```python
from build123d import *

# Parameters (mm, degrees)
EXTRUDE_1_DEPTH     = 35
SKETCH_7_W          = 12
SKETCH_7_H          = 6.5
EXTRUDE_3_DEPTH     = 4
CUT_EXTRUDE_1_REACH = 5
SKETCH_2_R          = 1.5
CUT_EXTRUDE_2_DEPTH = 28.8
SKETCH_6_W          = 12
SKETCH_6_H          = 5.977376498
SKETCH_6_R          = 1.5
EXTRUDE_2_DEPTH     = 4
CUT_EXTRUDE_3_REACH = 29.964
SKETCH_9_R          = 1.5
FILLET_1_R          = 3
FILLET_2_R          = 2
MM_CLEARANCE_1_D    = 3


with BuildPart() as part:
    # 草图1 → 凸台-拉伸1 (new body)
    with BuildSketch(Plane.XY):
        Polygon((-25.8, 21.661752689), (-25.8, -6.245255474), (3, -6.245255474), (3, 21.718248175), (0, 21.718248175), (0, -3.245255474), (-22.8, -3.245255474), (-22.8, 21.718248175), (-25.8, 21.718248175), align=None)
    extrude(amount=EXTRUDE_1_DEPTH)

    # 草图7 → 凸台-拉伸3 (add)
    with BuildSketch(Plane(origin=(0, -3.245255474, 0), x_dir=(1, 0, 0), z_dir=(0, 1, 0))):
        with Locations((-11.4, -3.272623502)):
            Rectangle(SKETCH_7_W, SKETCH_7_H)
    extrude(amount=EXTRUDE_3_DEPTH)

    # 草图2 → 切除-拉伸1 (cut, up to next)
    with BuildSketch(Plane(origin=(0, -3.245255474, 0), x_dir=(1, 0, 0), z_dir=(0, 1, 0)), mode=Mode.PRIVATE) as cut_extrude_1_sk1:
        with Locations((-11.4, -4.329564509)):
            Circle(SKETCH_2_R)
    cut_extrude_1_tool1 = extrude(cut_extrude_1_sk1.sketch, amount=-CUT_EXTRUDE_1_REACH, mode=Mode.PRIVATE) & part.part
    add(cut_extrude_1_tool1.solids().sort_by_distance((-11.4, -3.245255, 4.329565))[0], mode=Mode.SUBTRACT)
    # 草图2 → 切除-拉伸1 (cut, up to next)
    with BuildSketch(Plane(origin=(0, -3.245255474, 0), x_dir=(1, 0, 0), z_dir=(0, 1, 0)), mode=Mode.PRIVATE) as cut_extrude_1_sk2:
        with Locations((-11.4, -31.529564509)):
            Circle(SKETCH_2_R)
    cut_extrude_1_tool2 = extrude(cut_extrude_1_sk2.sketch, amount=-CUT_EXTRUDE_1_REACH, mode=Mode.PRIVATE) & part.part
    add(cut_extrude_1_tool2.solids().sort_by_distance((-11.4, -3.245255, 31.529565))[0], mode=Mode.SUBTRACT)
    # 草图2 → 切除-拉伸1 (cut, up to next)
    with BuildSketch(Plane(origin=(0, -3.245255474, 0), x_dir=(1, 0, 0), z_dir=(0, 1, 0)), mode=Mode.PRIVATE) as cut_extrude_1_sk3:
        with BuildLine():
            Line((-14.65, -18), (-14.65, -16.99341649))
            ThreePointArc((-14.65, -16.99341649), (-11.4, -6.5), (-8.15, -16.99341649))
            Line((-8.15, -16.99341649), (-8.15, -18))
            ThreePointArc((-8.15, -18), (-11.4, -21.25), (-14.65, -18))
        make_face()
    cut_extrude_1_tool3 = extrude(cut_extrude_1_sk3.sketch, amount=-CUT_EXTRUDE_1_REACH, mode=Mode.PRIVATE) & part.part
    add(cut_extrude_1_tool3.solids().sort_by_distance((-11.4, -3.245255, 13.308508))[0], mode=Mode.SUBTRACT)

    # 草图5 → 切除-拉伸2 (cut)
    with BuildSketch(Plane.ZY.offset(25.8)):
        with BuildLine():
            Line((0, 6.647160947), (0, 21.718248175))
            Line((0, 21.718248175), (21.134010141, 21.718248175))
            Line((21.134010141, 21.718248175), (2.843364957, 11.158139254))
            ThreePointArc((2.843364957, 11.158139254), (0.770155132, 9.313321556), (0, 6.647160947))
        make_face()
    extrude(amount=-CUT_EXTRUDE_2_DEPTH, mode=Mode.SUBTRACT)

    # 草图6 → 凸台-拉伸2 (add)
    with BuildSketch(Plane(origin=(0, -3.245255474, 0), x_dir=(1, 0, 0), z_dir=(0, 1, 0))):
        with Locations((-11.353661672, -32.011311751)):
            Rectangle(SKETCH_6_W, SKETCH_6_H)
        with Locations((-11.4, -31.529564509)):
            Circle(SKETCH_6_R, mode=Mode.SUBTRACT)
    extrude(amount=EXTRUDE_2_DEPTH)

    # 草图9 → 切除-拉伸3 (cut, up to next)
    with BuildSketch(Plane.XZ.offset(6.245255474), mode=Mode.PRIVATE) as cut_extrude_3_sk1:
        with Locations((-11.4, 4.329564509)):
            Circle(SKETCH_9_R)
    cut_extrude_3_tool1 = extrude(cut_extrude_3_sk1.sketch, amount=-CUT_EXTRUDE_3_REACH, mode=Mode.PRIVATE) & part.part
    add(cut_extrude_3_tool1.solids().sort_by_distance((-11.4, -6.245255, 4.329565))[0], mode=Mode.SUBTRACT)

    # 圆角1
    fillet_1_edges = [part.edges().sort_by_distance(p)[0] for p in [
        (-22.8, -3.245255474, 17.5),
        (0, -3.245255474, 17.5),
    ]]
    fillet(fillet_1_edges, radius=FILLET_1_R)

    # 圆角2
    fillet_2_edges = [part.edges().sort_by_distance(p)[0] for p in [
        (-5.4, -3.245255474, 3.272623502),
        (-17.4, -3.245255474, 3.272623502),
        (-5.353661672, -3.245255474, 32.011311751),
        (-17.353661672, -3.245255474, 32.011311751),
    ]]
    fillet(fillet_2_edges, radius=FILLET_2_R)

    # 大小mm Clearance 暗销孔1 (through all)
    with Locations(Plane(origin=(3, -125.31519419, 113.107396439), x_dir=(0, 0.022253058, -0.99975237), z_dir=(1, 0, 0))):
        with Locations((88.938953066, 135.227377046), (101.942467158, 126.647536361), (127.53759353, 125.598807912), (135.454300746, 124.4473971)):
            Hole(MM_CLEARANCE_1_D / 2)


solid = part.part
```
Can you work these out from the model? Positions are in its coordinate system, mm. A direction names the side the tool comes from. Coordinates: 2 decimals unless noted, no trailing zeros. Order: outer loops, then holes, each group sorted by start corner. A loop starts at its lowest first (then second) coordinate and runs counter-clockwise, first axis right, second up. Notation, with made-up numbers: (10.25, -23.5) -> (66.25, -23.5) arc R30 cw to (66.25, 7.5) -> close; hole circle Ø4 at (-12, 42). An arc over 180 degrees is marked (long way). Write each question's results on one line, items separated by ' | '.
Item 1: Which directions (+Z, -Z, +X, -X, +Y, -Y) give clear straight access to the entire face, cutting with the end or side of a thin tool? Please do faces 1 (the face through (-17.354, 0, 32)), 2 (the face through (-9, -3.245, 21)), 3 (the face through (-21.9, -2.39, 17.74)), 4 (the face through (-4.799, -2.675, 3.227)), 5 (the face through (-11.33, -4.72, 21.25)).
Results are:
face 1: +Z, +Y | face 2: +Y | face 3: +Z, -Z, +Y | face 4: -Z, +Y | face 5: +Y, -Y
Item 2: If I drill on line 1 along Z through (x, y) = (-11.4, -1); line 2 along X through (y, z) = (6.75, 28.5); line 3 along Z through (x, y) = (-7.75, -1.5), over which ranges is the centre line in solid material (lowest first)?
Results are:
line 1: 0.02 to 2.83, 5.83 to 6.52, 29.02 to 30.03, 33.03 to 35 | line 2: -25.8 to -22.8, 0 to 3 | line 3: 0.02 to 6.52, 29.02 to 35
Item 3: I'm going to push flat-ended pins straight in: pin 1 Ø2 at (x, y) = (-9.5, -0.5) entering from -Z; pin 2 Ø4 at (x, z) = (-3, 8.5) entering from +Y; pin 3 Ø1 at (x, z) = (-6, 14.5) entering from +Y. Where does each tip first touch, or does it pass through?
Results are:
pin 1: z = 0.02 | pin 2: y = -2.48 | pin 3: y = -3.25
Item 4: I want a section at C-C, the plane z = 17.5. Write out the boundary of the cut face in (x, y), then the cut area to 3 significant figures.
Results are:
outline: (-25.8, -6.25) -> (-14.65, -6.25) -> (-14.65, -3.25) -> (-19.8, -3.25) arc R3 cw to (-22.8, -0.25) -> (-22.8, 19.62) -> (-25.8, 19.62) -> close; (-8.15, -6.25) -> (3, -6.25) -> (3, 19.62) -> (0, 19.62) -> (0, -0.25) arc R3 cw to (-3, -3.25) -> (-8.15, -3.25) -> close | area: 208 mm²
Item 5: I want a section at D-D, the plane y = 18.25. Write out the boundary of the cut face in (x, z).
Results are:
outline: (-25.8, 15.13) -> (-22.8, 15.13) -> (-22.8, 35) -> (-25.8, 35) -> close; (0, 15.13) -> (3, 15.13) -> (3, 35) -> (0, 35) -> close
Item 6: I want a section at B-B, the plane y = -0.75. Write out the boundary of the cut face in (x, z).
Results are:
outline: (-25.8, 0) -> (-22.76, 0) -> (-22.76, 35) -> (-25.8, 35) -> close; (-17.4, 0.02) -> (-5.4, 0.02) -> (-5.4, 6.52) -> (-17.4, 6.52) -> close; (-17.35, 29.02) -> (-5.35, 29.02) -> (-5.35, 35) -> (-17.35, 35) -> close; (-0.04, 0) -> (3, 0) -> (3, 35) -> (-0.04, 35) -> close; hole circle Ø3 at (-11.4, 4.33); hole circle Ø3 at (-11.4, 31.53)
Item 7: I want a section at A-A, the plane x = -11.4. Count the separate pieces of the cut face and the enclosed holes in it, then the cut area to 3 significant figures.
Results are:
separate pieces: 4 | enclosed holes: 0 | area: 68.7 mm²
Item 8: If we mould it in two halves opening along Y, with no side actions, what happens to faces 6 (the face through (1.479, 9.347, 0.791)), 7 (the face through (-24.32, 2.68, 12.8)), 8 (the face through (-17.4, 0, 3))? For each: +Y half, -Y half, draft (parallel to the pull), parting line (faces both ways), or undercut.
Results are:
face 6: +Y half | face 7: undercut | face 8: draft
